Autodesk Inventor part; units mm, degrees
ref_plane "YZ Plane" through (0, 0, 0) normal (1, 0, 0) x (0, 1, 0)
ref_plane "XZ Plane" through (0, 0, 0) normal (0, 1, 0) x (-1, 0, 0)
ref_plane "XY Plane" through (0, 0, 0) normal (0, 0, 1) x (1, 0, 0)
sketch "スケッチ1" plane through (0, 0, 0) normal (0, 0, 1) x (1, 0, 0)
  line L0 (0, 0) -> (26, 0)
  line L1 (26, 0) -> (26, 18)
  line L2 (26, 18) -> (0, 18)
  line L3 (0, 18) -> (0, 0)
  dimension "d0" = 26
  dimension "d1" = 18
extrude "押し出し1" add sketch "スケッチ1" along normal blind 1.6
sketch "スケッチ2" plane through (0, 0, 1.6) normal (0, 0, 1) x (1, 0, 0)
  line L0 (0, 0) -> (26, 0)
  line L1 (26, 0) -> (26, 18)
  line L2 (26, 18) -> (0, 18)
  line L3 (0, 18) -> (0, 0)
  line L4 (23.5, 2.5) -> (2.5, 2.5)
  line L5 (2.5, 2.5) -> (2.5, 15.5)
  line L6 (2.5, 15.5) -> (23.5, 15.5)
  line L7 (23.5, 15.5) -> (23.5, 2.5)
  dimension "d4" = 2.5
hole "穴1" at (23.5, 15.5, 1.6) at (23.5, 2.5, 1.6) at (2.5, 2.5, 1.6) at (2.5, 15.5, 1.6) direction (0, 0, -1) diameter 2.2 end through all
fillet "フィレット1" radius 1 4 edges at (0, 0, 0.8) (26, 0, 0.8) (0, 18, 0.8) (26, 18, 0.8)
sketch "スケッチ4" plane through (0, 0, 1.6) normal (0, 0, 1) x (1, 0, 0)
  circle A0 centre (2.5, 2.5) radius 1.1
  circle A1 centre (23.5, 15.5) radius 1.1
  circle A2 centre (23.5, 2.5) radius 1.1
  circle A3 centre (2.5, 15.5) radius 1.1
  arc A4 (26, 17) -> (25, 18) centre (25, 17) ccw
  line L0 (25, 18) -> (1, 18)
  arc A5 (1, 18) -> (0, 17) centre (1, 17) ccw
  line L1 (0, 17) -> (0, 1)
  arc A6 (0, 1) -> (1, 0) centre (1, 1) ccw
  line L2 (1, 0) -> (25, 0)
  arc A7 (25, 0) -> (26, 1) centre (25, 1) ccw
  line L3 (26, 1) -> (26, 17)
  line L4 (15, 15.3) -> (21, 15.3)
  line L5 (21, 15.3) -> (21, 9.3)
  line L6 (21, 9.3) -> (15, 9.3)
  line L7 (15, 9.3) -> (15, 15.3)
  line L8 (26, 1) -> (26, 17)
  line L9 (26, 9) -> (14.7, 9)
  line L10 (15, 2.7) -> (21, 2.7)
  line L11 (21, 2.7) -> (21, 8.7)
  line L12 (21, 8.7) -> (15, 8.7)
  line L13 (15, 8.7) -> (15, 2.7)
  line L14 (14.7, 9) -> (14.7, 10.3555)
  line L15 (14.4, 15.3) -> (8.4, 15.3)
  line L16 (8.4, 15.3) -> (8.4, 9.3)
  line L17 (8.4, 9.3) -> (14.4, 9.3)
  line L18 (14.4, 9.3) -> (14.4, 15.3)
  line L19 (14.4, 8.7) -> (14.4, 2.7)
  line L20 (14.4, 2.7) -> (8.4, 2.7)
  line L21 (8.4, 8.7) -> (14.4, 8.7)
  line L22 (8.4, 2.7) -> (8.4, 8.7)
  point P0 (0, 0)
  dimension "d24" = 6
  dimension "d25" = 6
  dimension "d26" = 0.6
  dimension "d27" = 0.6
  dimension "d28" = 5
extrude "押し出し2" add sketch "スケッチ4" along normal blind 8.3 contours L4 L5 L6 L7 | L13 L12 L11 L10 | L18 L17 L16 L15 | L19 L20 L22 L21
sketch "スケッチ6" plane through (0, 0, 1.6) normal (0, 0, 1) x (1, 0, 0)
  line L0 (0, 17) -> (0, 1)
  line L1 (0, 9) -> (6.7, 9)
  line L2 (6.7, 9) -> (6.7, 11.5)
  circle A0 centre (6.7, 11.5) radius 0.8483
  circle A1 centre (6.7, 9) radius 0.8884
  circle A2 centre (6.7, 6.5) radius 0.8483
  circle A3 centre (6.7, 9) radius 0.8884
  point P0 (0, 0)
  dimension "d33" = 6.7
  dimension "d34" = 2.5
  dimension "d35" = 0
hole "穴3" at (6.7, 11.5, 1.6) at (6.7, 9, 1.6) at (6.7, 9, 1.6) at (6.7, 6.5, 1.6) direction (0, 0, -1) diameter 1 end through all
sketch "スケッチ8" plane through (0, 0, 1.6) normal (0, 0, 1) x (1, 0, 0)
  circle A0 centre (6.7, 9) radius 0.5
  circle A1 centre (6.7, 11.5) radius 0.5
  circle A2 centre (6.7, 6.5) radius 0.5
  line L0 (14.4, 15.3) -> (14.4, 9.3)
  line L1 (14.4, 9.3) -> (8.4, 9.3)
  line L2 (8.4, 9.3) -> (8.4, 15.3)
  line L3 (8.4, 15.3) -> (14.4, 15.3)
  line L4 (21, 15.3) -> (21, 9.3)
  line L5 (21, 9.3) -> (15, 9.3)
  line L6 (15, 9.3) -> (15, 15.3)
  line L7 (15, 15.3) -> (21, 15.3)
  line L8 (21, 8.7) -> (21, 2.7)
  line L9 (21, 2.7) -> (15, 2.7)
  line L10 (15, 2.7) -> (15, 8.7)
  line L11 (15, 8.7) -> (21, 8.7)
  line L12 (14.4, 8.7) -> (14.4, 2.7)
  line L13 (14.4, 2.7) -> (8.4, 2.7)
  line L14 (8.4, 2.7) -> (8.4, 8.7)
  line L15 (8.4, 8.7) -> (14.4, 8.7)
  circle A3 centre (2.5, 2.5) radius 1.1
  circle A4 centre (23.5, 15.5) radius 1.1
  circle A5 centre (23.5, 2.5) radius 1.1
  circle A6 centre (2.5, 15.5) radius 1.1
  arc A7 (26, 17) -> (25, 18) centre (25, 17) ccw
  line L16 (25, 18) -> (1, 18)
  arc A8 (1, 18) -> (0, 17) centre (1, 17) ccw
  line L17 (0, 17) -> (0, 1)
  arc A9 (0, 1) -> (1, 0) centre (1, 1) ccw
  line L18 (1, 0) -> (25, 0)
  arc A10 (25, 0) -> (26, 1) centre (25, 1) ccw
  line L19 (26, 1) -> (26, 17)
  line L20 (6.7, 6.5) -> (6.7, 4)
  circle A11 centre (6.7, 4) radius 0.5842
  point P0 (0, 0)
  dimension "d44" = 2.5
hole "穴4" at (6.7, 4, 1.6) direction (0, 0, -1) diameter 1 end through all
properties part number "中継ハブ" material "GFRC"
Can you work these out from the model? Positions are in its coordinate system, mm. A direction names the side the tool comes from. Coordinates: 2 decimals unless noted, no trailing zeros. Write each loop counter-clockwise with the first axis right and the second up, starting at its lowest first coordinate (ties: lowest second). Pieces come first, ordered by that corner, then holes. Notation, with made-up numbers: (27, 64.5) - (63, 64.5) arc R32 cw to (63, 92.5) - close; hole circle Ø7 at (3.5, 76.25). An arc over 180 degrees is marked (long way). Return JSON: item names as keys, results as strings. Group by question number.
Item 1: If we section it at C-C (x = 2.5): Write out the boundary of the cut face in (y, z), then the cut area to 3 significant figures.
Item 2: Which directions (+Z, -Z, +X, -X, +Y, -Y) give clear straight access to the entire face, cutting with the end or side of a thin tool? Please do faces 1 (the face through (11, 2.7, 6)), 2 (the face through (14.4, 12, 6)), 3 (the face through (8.4, 6, 6)).
Item 3: If we section it at B-B (y = 4): Write out the boundary of the cut face in (x, z), then the cut area to 3 significant figures.
Item 4: We'd pull the mould along X, two halves only. Please class faces 4 (the face through (11, 12, 9.9)), 5 (the face through (0.301, 17.715, 0.811)), 6 (the face through (7.188, 4.108, 0.789)): pulls with the +X half, pulls with the -X half, needs draft (parallel to the pull), parting line crosses it, or undercut.
Item 5: Please list where these lines run through material, in increasing order: probe 1 along Y at (x, z) = (2.5, 0.5); probe 2 along X at (y, z) = (15.5, 0.55); probe 3 along Y at (x, z) = (6.7, 0.55).
Item 6: If we section it at A-A (x = 6.7): Write out the boundary of the cut face in (y, z).
Item 7: If we section it at D-D (z = 2.5): Write out the boundary of the cut face in (x, y), then the cut area to 3 significant figures.
Item 8: I'm going to push flat-ended pins straight in: pin 1 Ø1 at (y, z) = (14, 6.5) entering from +X; pin 2 Ø3 at (y, z) = (6, 4) entering from -X; pin 3 Ø3 at (x, z) = (11, 6) entering from -Y; pin 4 Ø2 at (x, y) = (23.5, 2.5) entering from -Z. Where does each tip first touch, or does it pass through?
Return value:
{
 "1": {"outline": "(0, 0) - (1.4, 0) - (1.4, 1.6) - (0, 1.6) - close; (3.6, 0) - (14.4, 0) - (14.4, 1.6) - (3.6, 1.6) - close; (16.6, 0) - (18, 0) - (18, 1.6) - (16.6, 1.6) - close", "area": "21.8 mm^2"},
 "2": {"face 1": "+Z, +X, -X, -Y", "face 2": "+Z, +Y, -Y", "face 3": "+Z, -X, +Y, -Y"},
 "3": {"outline": "(0, 0) - (6.2, 0) - (6.2, 1.6) - (0, 1.6) - close; (7.2, 0) - (26, 0) - (26, 1.6) - (21, 1.6) - (21, 9.9) - (15, 9.9) - (15, 1.6) - (14.4, 1.6) - (14.4, 9.9) - (8.4, 9.9) - (8.4, 1.6) - (7.2, 1.6) - close", "area": "140 mm^2"},
 "4": {"face 4": "needs draft", "face 5": "pulls with the -X half", "face 6": "undercut"},
 "5": {"probe 1": "y = 0 to 1.4, 3.6 to 14.4, 16.6 to 18", "probe 2": "x = 0 to 1.4, 3.6 to 22.4, 24.6 to 26", "probe 3": "y = 0 to 3.5, 4.5 to 6, 7 to 8.5, 9.5 to 11, 12 to 18"},
 "6": {"outline": "(0, 0) - (3.5, 0) - (3.5, 1.6) - (0, 1.6) - close; (4.5, 0) - (6, 0) - (6, 1.6) - (4.5, 1.6) - close; (7, 0) - (8.5, 0) - (8.5, 1.6) - (7, 1.6) - close; (9.5, 0) - (11, 0) - (11, 1.6) - (9.5, 1.6) - close; (12, 0) - (18, 0) - (18, 1.6) - (12, 1.6) - close"},
 "7": {"outline": "(8.4, 2.7) - (14.4, 2.7) - (14.4, 8.7) - (8.4, 8.7) - close; (8.4, 9.3) - (14.4, 9.3) - (14.4, 15.3) - (8.4, 15.3) - close; (15, 2.7) - (21, 2.7) - (21, 8.7) - (15, 8.7) - close; (15, 9.3) - (21, 9.3) - (21, 15.3) - (15, 15.3) - close", "area": "144 mm^2"},
 "8": {"pin 1": "stops at x = 21", "pin 2": "stops at x = 8.4", "pin 3": "stops at y = 2.7", "pin 4": "passes through"}
}
